Input: part model. Units: mm. Frame: model coordinates. Face numbers are marked on the shaded views. A direction names the side the tool comes from. Coordinates: 2 decimals unless noted, no trailing zeros. Loops run counter-clockwise (first coordinate to the right, second up) from the corner with the lowest first, then second, coordinate; pieces in that order, holes last.
```python
from build123d import *

# Parameters (mm, degrees)
SKETCH1_W               = 20
SKETCH1_H               = 45
SKETCH1_R               = 5
BOSS_EXTRUDE1_DEPTH     = 75
SKETCH2_R               = 3.25
CUT_EXTRUDE1_DEPTH      = 90.721792225
SKETCH5_R               = 6
SKETCH5_R_2             = 2.75
BOSS_EXTRUDE3_DEPTH     = 9
CUT_EXTRUDE2_REACH      = 91.722
SKETCH6_R               = 2.75
BOSS_EXTRUDE4_DEPTH     = 5
CUT_EXTRUDE3_REACH      = 94.603
CUT_EXTRUDE3_END_RADIUS = 6
SKETCH9_R               = 1.8


with BuildPart() as part:
    # Sketch1 → Boss-Extrude1 (new body)
    with BuildSketch(Plane(origin=(0, 0, 0), x_dir=(0, 0, -1), z_dir=(1, 0, 0))):
        with Locations((10, 22.5)):
            Rectangle(SKETCH1_W, SKETCH1_H)
        with Locations((10, 35)):
            Circle(SKETCH1_R, mode=Mode.SUBTRACT)
        with Locations((10, 10)):
            Circle(SKETCH1_R, mode=Mode.SUBTRACT)
    extrude(amount=BOSS_EXTRUDE1_DEPTH)

    # Sketch2 → Cut-Extrude1 (cut, through all)
    with BuildSketch(Plane.XY):
        with Locations((10, 22.5)):
            Circle(SKETCH2_R)
        with Locations((65, 22.5)):
            Circle(SKETCH2_R)
    extrude(amount=-CUT_EXTRUDE1_DEPTH, mode=Mode.SUBTRACT)

    # Sketch4 → Cut-Revolve1 (revolve, cut)
    with BuildSketch(Plane.XY.offset(-10), mode=Mode.PRIVATE) as cut_revolve1_sk:
        Polygon((12, 40), (13.732050808, 41), (61.267949192, 41), (63, 40), align=None)
    cut_revolve1 = revolve(cut_revolve1_sk.sketch.rotate(Axis((75, 35, -10), (-1, 0, 0)), 90), axis=Axis((75, 35, -10), (-1, 0, 0)), mode=Mode.SUBTRACT)

    # Mirror1: Cut-Revolve1 across plane
    add(cut_revolve1.mirror(Plane.ZX.offset(22.5)), mode=Mode.SUBTRACT)

    # Sketch5 → Boss-Extrude3 (add)
    with BuildSketch(Plane.ZY):
        with Locations((-10, 22.5)):
            Circle(SKETCH5_R)
        with Locations((-10, 22.5)):
            Circle(SKETCH5_R_2, mode=Mode.SUBTRACT)
    extrude(amount=BOSS_EXTRUDE3_DEPTH)

    # Sketch6 → Cut-Extrude2 (cut, up to next)
    with BuildSketch(Plane.ZY, mode=Mode.PRIVATE) as cut_extrude2_sk1:
        with Locations((-10, 22.5)):
            Circle(SKETCH6_R)
    cut_extrude2_tool1 = extrude(cut_extrude2_sk1.sketch, amount=-CUT_EXTRUDE2_REACH, mode=Mode.PRIVATE) & part.part
    add(cut_extrude2_tool1.solids().sort_by_distance((0, 22.5, -10))[0], mode=Mode.SUBTRACT)

    # Sketch8 → Boss-Extrude4 (add, symmetric)
    with BuildSketch(Plane.XY.offset(-10)):
        Polygon((52.757359313, 45), (58.257359313, 50.5), (66.242640687, 50.5), (71.742640687, 45), (65, 45), (65, 47.5), (59.5, 47.5), (59.5, 45), align=None)
    extrude(amount=BOSS_EXTRUDE4_DEPTH, both=True)

    # Cut-Extrude3: up to this cylinder (the profile starts outside it)
    cut_extrude3_end = Plane(origin=(62.25, 35, -10), z_dir=(1, 0, 0)) * Cylinder(CUT_EXTRUDE3_END_RADIUS, 202.206, mode=Mode.PRIVATE)
    # Sketch9 → Cut-Extrude3 (cut, up to the surface)
    with BuildSketch(Plane(origin=(0, 50.5, 0), x_dir=(1, 0, 0), z_dir=(0, 1, 0)), mode=Mode.PRIVATE) as cut_extrude3_sk1:
        with Locations(Location((62.25, 10, 0), (0, 0, 270))):
            Circle(SKETCH9_R)
    cut_extrude3_tool1 = extrude(cut_extrude3_sk1.sketch, amount=-CUT_EXTRUDE3_REACH, mode=Mode.PRIVATE) - cut_extrude3_end
    add(cut_extrude3_tool1.solids().sort_by_distance((62.25, 50.5, -10))[0], mode=Mode.SUBTRACT)


solid = part.part
```
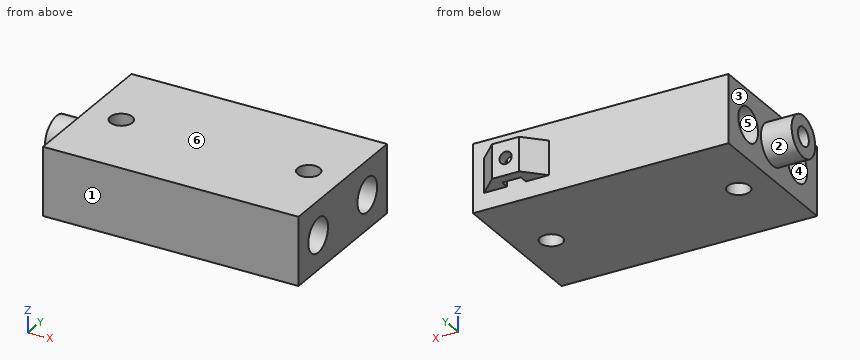
Item 1: Mould query, pull axis Z, two halves, no side actions, for the marked faces 3, 4, 5 and 6. Classes: +Z half, -Z half, draft (parallel to the pull), parting line (faces both ways), or undercut.
Result:
face 3: draft
face 4: undercut
face 5: undercut
face 6: +Z half
Item 2: Section query A-A (y = 10). Output: boundary loops of the cut face in (x, z), then the cut area to 3 significant figures.
Result:
outline: (0, -20) - (75, -20) - (75, -15) - (63, -15) - (61.27, -16) - (13.73, -16) - (12, -15) - (0, -15) - close; (0, -5) - (12, -5) - (13.73, -4) - (61.27, -4) - (63, -5) - (75, -5) - (75, 0) - (0, 0) - close
area: 651 mm2
Item 3: Section query B-B (y = 22.5). Output: boundary loops of the cut face in (x, z), then the cut area to 3 significant figures.
Result:
outline: (-9, -16) - (0, -16) - (0, -20) - (6.75, -20) - (6.75, -12.75) - (-9, -12.75) - close; (-9, -7.25) - (6.75, -7.25) - (6.75, 0) - (0, 0) - (0, -4) - (-9, -4) - close; (13.25, -20) - (61.75, -20) - (61.75, 0) - (13.25, 0) - close; (68.25, -20) - (75, -20) - (75, 0) - (68.25, 0) - close
area: 1,260 mm2
Item 4: Section query C-C (z = -10). Count the separate pieces of the cut face and the enclosed holes in it, then the cut area to 3 significant figures.
Result:
separate pieces: 4
enclosed holes: 1
area: 1,670 mm2
Item 5: Contact query for flat-ended pins moving along their axis: P1, Ø4.5, axis at x = 66, y = 49, coming from the -Z side; P2, Ø8, axis at x = 33, z = -6.5, coming from the +Y side; P3, Ø8, axis at y = 10, z = -10, coming from the +X side; P4, Ø0.8, axis at y = 46, z = -12, coming from the +X side. Output: stop coordinate, or through.
Result:
P1: stops at z = -15
P2: stops at y = 45
P3: passes through
P4: stops at x = 71.14
Item 6: Line query: L1, parallel to X at y = 42.7, z = -10; L2, parallel to Y at x = -6.75, z = -10; L3, parallel to Y at x = 26.5, z = -8. Output: solid intervals per line, ascending.
Result:
L1: x = 0 to 60.45, 64.05 to 75
L2: y = 16.5 to 19.75, 25.25 to 28.5
L3: y = 0 to 4.34, 15.66 to 29.34, 40.66 to 45
Item 7: Reachability of the marked faces 1 and 2 from +Z, -Z, +X, -X, +Y, -Y: full face, straight path, thin tool, end or side. Return the list, or none.
Result:
face 1: +Z, -Z, +X, -X, -Y
face 2: -X
